```python
from build123d import *

# Parameters (mm, degrees)
F0_W      = 124.8
F0_H      = 81
F1_DEPTH  = 33
F2_W      = 122.5
F2_H      = 78.7
F3_DEPTH  = 3
F4_W      = 120.8
F4_H      = 77
F5_DEPTH  = 34
F6_W      = 10
F6_H      = 10
F7_DEPTH  = 24.4
F8_R      = 1.5
F9_DEPTH  = 4.8
F10_W     = 26
F10_H     = 46
F10_W_2   = 20
F10_H_2   = 12.8
F10_W_3   = 12.8
F10_H_3   = 30.7
F11_DEPTH = 2.001
F12_R     = 3
F13_DEPTH = 4
F14_R     = 1.5
F15_DEPTH = 4.8
F16_W     = 12
F16_H     = 57
F17_DEPTH = 6
F18_R     = 1.5
F19_DEPTH = 4.8
F20_W     = 26
F20_H     = 16
F21_DEPTH = 6
F22_R     = 1.5
F23_DEPTH = 4.8
F24_R     = 5
F24_R_2   = 4
F25_DEPTH = 1
F27_DEPTH = 1
F28_R     = 4.25
F28_R_2   = 3.65
F29_DEPTH = 1


with BuildPart() as f1:
    # F0 (on Top) → F1 (new body)
    with BuildSketch(Plane.XY):
        Rectangle(F0_W, F0_H)
    extrude(amount=F1_DEPTH)

    # F2 (on face) → F3 (join)
    with BuildSketch(Plane.XY.offset(33)):
        Rectangle(F2_W, F2_H)
    extrude(amount=F3_DEPTH)

    # F4 (on face) → F5 (cut)
    with BuildSketch(Plane.XY.offset(36)):
        Rectangle(F4_W, F4_H)
    extrude(amount=-F5_DEPTH, mode=Mode.SUBTRACT)

    # F6 (on face) → F7 (join)
    with BuildSketch(Plane.XY.offset(2)):
        with Locations((-55.4, 33.5)):
            Rectangle(F6_W, F6_H)
        with Locations((-55.4, -33.5)):
            Rectangle(F6_W, F6_H)
        with Locations((55.4, -33.5)):
            Rectangle(F6_W, F6_H)
        with Locations((55.4, 33.5)):
            Rectangle(F6_W, F6_H)
    extrude(amount=F7_DEPTH)

    # F8 (on face) → F9 (cut)
    with BuildSketch(Plane.XY.offset(26.4)):
        with Locations((-55, 33.5)):
            Circle(F8_R)
        with Locations((-55, -33.5)):
            Circle(F8_R)
        with Locations((55, -33.5)):
            Circle(F8_R)
        with Locations((55, 33.5)):
            Circle(F8_R)
    extrude(amount=-F9_DEPTH, mode=Mode.SUBTRACT)

    # F10 (on face) → F11 (cut, through all)
    with BuildSketch(Plane.XY.offset(2)):
        with Locations((44.4, 4.5)):
            Rectangle(F10_W, F10_H)
        with Locations((23.4, -29.1)):
            Rectangle(F10_W_2, F10_H_2)
        with Locations((9.5, 0)):
            Rectangle(F10_W_3, F10_H_3)
    extrude(amount=-F11_DEPTH, mode=Mode.SUBTRACT)

    # F12 (on face) → F13 (join)
    with BuildSketch(Plane.XY.offset(2)):
        with Locations((24.4, 13.2)):
            Circle(F12_R)
        with Locations((-34.6, 13.2)):
            Circle(F12_R)
        with Locations((-34.6, -15.8)):
            Circle(F12_R)
        with Locations((24.4, -15.8)):
            Circle(F12_R)
        with Locations((-43.4, 31.5)):
            Circle(F12_R)
        with Locations((-43.4, 22.5)):
            Circle(F12_R)
        with Locations((-20.4, 31.5)):
            Circle(F12_R)
        with Locations((-5.4, 31.5)):
            Circle(F12_R)
        with Locations((11.6, 31.5)):
            Circle(F12_R)
    extrude(amount=F13_DEPTH)

    # F14 (on face) → F15 (cut)
    with BuildSketch(Plane.XY.offset(2)):
        with Locations((-34.6, -15.8)):
            Circle(F14_R)
        with Locations((24.4, -15.8)):
            Circle(F14_R)
        with Locations((-34.6, 13.2)):
            Circle(F14_R)
        with Locations((24.4, 13.2)):
            Circle(F14_R)
        with Locations((11.6, 31.5)):
            Circle(F14_R)
        with Locations((-5.4, 31.5)):
            Circle(F14_R)
        with Locations((-20.4, 31.5)):
            Circle(F14_R)
        with Locations((-43.4, 22.5)):
            Circle(F14_R)
        with Locations((-43.4, 31.5)):
            Circle(F14_R)
    extrude(amount=F15_DEPTH, mode=Mode.SUBTRACT)

    # F16 (on face) → F17 (join)
    with BuildSketch(Plane.XY.offset(2)):
        with Locations((-54.4, 0)):
            Rectangle(F16_W, F16_H)
    extrude(amount=F17_DEPTH)

    # F18 (on face) → F19 (cut)
    with BuildSketch(Plane.XY.offset(8)):
        with Locations((-54.4, 0)):
            Circle(F18_R)
    extrude(amount=-F19_DEPTH, mode=Mode.SUBTRACT)

    # F20 (on face) → F21 (join)
    with BuildSketch(Plane.XY.offset(2)):
        with Locations((-22.927424, -30.5)):
            Rectangle(F20_W, F20_H)
    extrude(amount=F21_DEPTH)

    # F22 (on face) → F23 (cut)
    with BuildSketch(Plane.XY.offset(8)):
        with Locations((-22.927424, -25)):
            Circle(F22_R)
        with Locations((-22.927424, -36)):
            Circle(F22_R)
    extrude(amount=-F23_DEPTH, mode=Mode.SUBTRACT)

    # F24 (on face) → F25 (join)
    with BuildSketch(Plane(origin=(0, 0, 0), x_dir=(1, 0, 0), z_dir=(0, 0, -1))):
        with Locations((47.4, 32.5)):
            Circle(F24_R)
        with Locations((47.4, 32.5)):
            Circle(F24_R_2, mode=Mode.SUBTRACT)
    extrude(amount=F25_DEPTH)

    # F26 (on face) → F27 (join)
    with BuildSketch(Plane(origin=(0, 0, 0), x_dir=(1, 0, 0), z_dir=(0, 0, -1))):
        Polygon((51.51844, 33.062976), (44.911735, 36.120117), (44.168741, 35.294835), (46.409786, 34.256469), (46.409786, 30.746656), (44.189125, 29.699225), (45.097549, 28.966295), (51.51844, 31.970277), align=None)
        Polygon((47.476035, 33.758733), (50.228067, 32.507077), (47.476035, 31.239656), align=None, mode=Mode.SUBTRACT)
    extrude(amount=F27_DEPTH)

    # F28 (on face) → F29 (join)
    with BuildSketch(Plane(origin=(0, 0, 0), x_dir=(1, 0, 0), z_dir=(0, 0, -1))):
        with Locations((19.612311, -19.062311)):
            Circle(F28_R)
        with Locations((-0.612311, 19.062311)):
            Circle(F28_R)
        with Locations((-0.612311, 19.062311)):
            Circle(F28_R_2, mode=Mode.SUBTRACT)
    extrude(amount=F29_DEPTH)


solid = f1.part
```
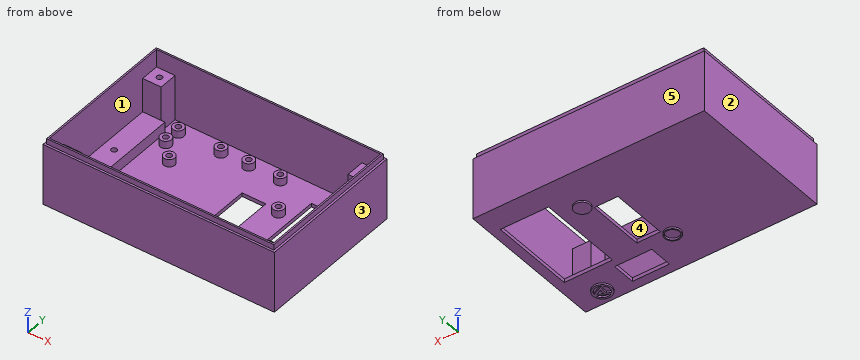
Geometry: final body of the model. Coordinates: model frame, mm. Face numbers are marked on the shaded views. A direction names the side the tool comes from. Give positions to 0.01 mm unless a question says otherwise; leave off trailing zeros. Loops run counter-clockwise (first coordinate to the right, second up) from the corner with the lowest first, then second, coordinate; pieces in that order, holes last. Notation, with made-up numbers: (-37, 21.5) -> (-20, 21.5) arc R30 cw to (-20, 57.5) -> close; hole circle Ø11 at (34.25, 65.25). An arc over 180 degrees is marked (long way). Use CSV: the item, a comma, the result in double quotes.
(1) Access query for the marked faces 4 and 5. Directions: +Z, -Z, +X, -X, +Y, -Y. A direction counts if a zero-diameter tool reaches every point of the face in a straight line with its end or side. Return the directions, or none.
From the geometry:
face 4,"+Z"
face 5,"+Z, -Z, +X, -X, +Y"
(2) First-contact query: P1, Ø12, axis at x = 17.5, y = -28, coming from the -Z side; P2, Ø2.5, axis at x = -34.6, y = 13.2, coming from the +Z side; P3, Ø6.5, axis at x = -6.5, y = 31, coming from the +Z side. Flat tips, straight axial feed; report the tip coordinate or a pass-through.
From the geometry:
P1,"z = 0"
P2,"z = 2"
P3,"z = 6"
(3) Cut plane A-A (x = 41). Output: boundary loops of the cut face in (y, z).
From the geometry:
outline,"(-40.5, 0) -> (-18.5, 0) -> (-18.5, 2) -> (-38.5, 2) -> (-38.5, 36) -> (-39.35, 36) -> (-39.35, 33) -> (-40.5, 33) -> close; (27.5, 0) -> (40.5, 0) -> (40.5, 33) -> (39.35, 33) -> (39.35, 36) -> (38.5, 36) -> (38.5, 2) -> (27.5, 2) -> close"
(4) Pull-direction query (X, two-part tool) for the marked faces 1, 2 and 3; classes: released by +X, released by -X, zero draft, split by the parting line, or undercut.
From the geometry:
face 1,"undercut"
face 2,"released by -X"
face 3,"released by +X"
(5) Ray query, line 1 along Y through (x, z) = (55, 23.8); line 2 along X through (y, z) = (0, 26); line 3 along Y through (x, z) = (-50, 31.5). Return the intervals inside material, ascending. Write a range as [from, to].
From the geometry:
line 1,"[-40.5, -35], [-32, -28.5], [28.5, 32], [35, 40.5]"
line 2,"[-62.4, -60.4], [60.4, 62.4]"
line 3,"[-40.5, -38.5], [38.5, 40.5]"
(6) Cut plane B-B (y = -7). Output: boundary loops of the cut face in (x, z).
From the geometry:
outline,"(-62.4, 0) -> (3.1, 0) -> (3.1, 2) -> (-48.4, 2) -> (-48.4, 8) -> (-60.4, 8) -> (-60.4, 36) -> (-61.25, 36) -> (-61.25, 33) -> (-62.4, 33) -> close; (15.9, 0) -> (31.4, 0) -> (31.4, 2) -> (15.9, 2) -> close; (57.4, 0) -> (62.4, 0) -> (62.4, 33) -> (61.25, 33) -> (61.25, 36) -> (60.4, 36) -> (60.4, 2) -> (57.4, 2) -> close"
(7) Cut plane D-D (z = 23.5). Output: boundary loops of the cut face in (x, y), plus the area to 3 significant figures.
From the geometry:
outline,"(-62.4, -40.5) -> (62.4, -40.5) -> (62.4, 40.5) -> (-62.4, 40.5) -> close; hole (-60.4, -28.5) -> (-50.4, -28.5) -> (-50.4, -38.5) -> (50.4, -38.5) -> (50.4, -28.5) -> (60.4, -28.5) -> (60.4, 28.5) -> (50.4, 28.5) -> (50.4, 38.5) -> (-50.4, 38.5) -> (-50.4, 28.5) -> (-60.4, 28.5) -> close; hole circle Ø3 at (-55, -33.5); hole circle Ø3 at (-55, 33.5); hole circle Ø3 at (55, -33.5); hole circle Ø3 at (55, 33.5)"
area,"1,180 mm^2"
(8) Cut plane C-C (z = 31.5). Output: boundary loops of the cut face in (x, y), plus the area to 3 significant figures.
From the geometry:
outline,"(-62.4, -40.5) -> (62.4, -40.5) -> (62.4, 40.5) -> (-62.4, 40.5) -> close; hole (-60.4, -38.5) -> (60.4, -38.5) -> (60.4, 38.5) -> (-60.4, 38.5) -> close"
area,"807 mm^2"
